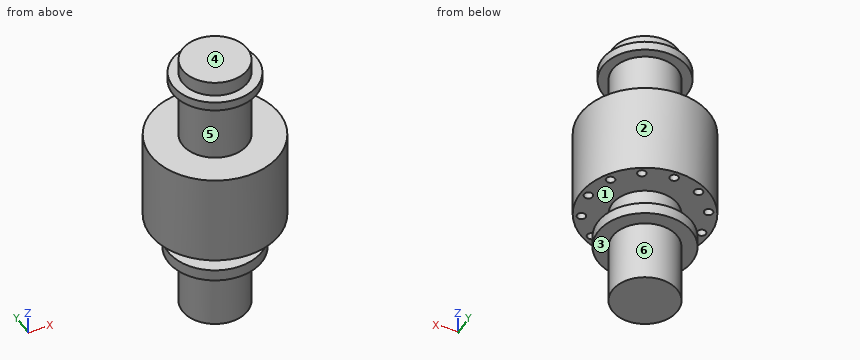
from build123d import *

# Parameters (mm, degrees)
SKETCH1_W          = 11.36904
SKETCH1_H          = 24.99995
SKETCH1_W_2        = 7.00024
SKETCH1_H_2        = 7.49935
SKETCH1_W_3        = 48.37938
SKETCH1_W_4        = 71.10476
SKETCH1_H_3        = 24.49957
SKETCH1_W_5        = 20.14982
SKETCH1_W_6        = 8.9916
SKETCH1_H_4        = 10.99947
SKETCH1_W_7        = 48.006
SKETCH2_R          = 3.3
CUT_EXTRUDE1_DEPTH = 9.525
CIRPATTERN2_COUNT  = 12


with BuildPart() as part:
    # Sketch1 → Revolve1 (revolve)
    with BuildSketch(Plane(origin=(0, 0, 0), x_dir=(0, 0, -1), z_dir=(1, 0, 0)), mode=Mode.PRIVATE) as revolve1_sk:
        with Locations((-101.8159, 12.499975)):
            Rectangle(SKETCH1_W, SKETCH1_H)
        with Locations((-92.63126, 12.499975)):
            Rectangle(SKETCH1_W_2, SKETCH1_H)
        with Locations((-92.63126, 28.749625)):
            Rectangle(SKETCH1_W_2, SKETCH1_H_2)
        with Locations((-64.94145, 12.499975)):
            Rectangle(SKETCH1_W_3, SKETCH1_H)
        with Locations((-5.19938, 12.499975)):
            Rectangle(SKETCH1_W_4, SKETCH1_H)
        with Locations((-5.19938, 37.249735)):
            Rectangle(SKETCH1_W_4, SKETCH1_H_3)
        with Locations((40.42791, 12.499975)):
            Rectangle(SKETCH1_W_5, SKETCH1_H)
        with Locations((54.99862, 12.499975)):
            Rectangle(SKETCH1_W_6, SKETCH1_H)
        with Locations((54.99862, 30.499685)):
            Rectangle(SKETCH1_W_6, SKETCH1_H_4)
        with Locations((83.49742, 12.499975)):
            Rectangle(SKETCH1_W_7, SKETCH1_H)
    revolve(revolve1_sk.sketch.rotate(Axis((0, 0, 107.50042), (0, 0, -1)), 180), axis=Axis((0, 0, 107.50042), (0, 0, -1)))

    # Sketch2 → Cut-Extrude1 (cut)
    with BuildSketch(Plane(origin=(0, 0, -30.353), x_dir=(-1, 0, 0), z_dir=(0, 0, -1))):
        with Locations(Location((0, 43.561, 0), (0, 0, 90))):
            Circle(SKETCH2_R)
    cut_extrude1 = extrude(amount=-CUT_EXTRUDE1_DEPTH, mode=Mode.SUBTRACT)

    # CirPattern2: Cut-Extrude1 ×12 about axis
    cirpattern2_axis = Axis((0, 0, 0), (0, 0, 1))
    for i in range(1, CIRPATTERN2_COUNT):
        add(cut_extrude1.rotate(cirpattern2_axis, i * 360 / CIRPATTERN2_COUNT), mode=Mode.SUBTRACT)


solid = part.part
Could you check a few things on this model? Use its own coordinates, in mm. Face numbers are marked on the shaded views. A direction names the side the tool comes from. Give positions to 0.01 mm unless a question says otherwise; leave off trailing zeros. Write each loop counter-clockwise with the first axis right and the second up, starting at its lowest first coordinate (ties: lowest second). Pieces come first, ordered by that corner, then holes. Notation, with made-up numbers: (-21, 15) -> (26, 15) arc R9 ccw to (26, 22) -> close; hole circle Ø2 at (-7.5, 84). An arc over 180 degrees is marked (long way). Answer as CSV lines item,"result". Start each with the question number.
(1) Which directions (+Z, -Z, +X, -X, +Y, -Y) give clear straight access to the entire face, cutting with the end or side of a thin tool? Please do the marked faces 4, 5 and 6.
(2) If we mould it in two halves opening along Z, with no side actions, what happens to the marked faces 1, 2 and 3? For each: +Z half, -Z half, draft (parallel to the pull), parting line (faces both ways), or undercut.
(3) Please list where these lines run through material, in increasing order: line 1 (Z direction, x = 6, y = -25.5); line 2 (X direction, y = 37, z = -28); line 3 (Z direction, x = -11, y = 40).
(4) If we section it at B-B, the plane y = 30: Write out the boundary of the cut face in (x, z).
(5) If we section it at C-C, the plane x = 7: Write out the boundary of the cut face in (y, z), and give its area (3 significant figures).
(6) I'm going to push flat-ended pins straight in: pin 1 Ø1 at (y, z) = (34.5, 23.5) entering from +X (3 decimals); pin 2 Ø3 at (y, z) = (-2.5, 21.5) entering from -X; pin 3 Ø12 at (x, z) = (-21, -32.5) entering from -Y; pin 4 Ø5 at (x, y) = (-26, 8.5) entering from +Z. Where does each tip first touch, or does it pass through?
(7) If we section it at A-A, the plane x = 29: Write out the boundary of the cut face in (y, z).
Answer list:
1,face 4,"+Z, +X, -X, +Y, -Y"
1,face 5,"none"
1,face 6,"-Z"
2,face 1,"undercut"
2,face 2,"draft"
2,face 3,"-Z half"
3,line 1,"-59.49 to -50.5, -30.35 to 40.75, 89.13 to 96.13"
3,line 2,"-32.88 to -25, -18.56 to 18.56, 25 to 32.88"
3,line 3,"-30.35 to 40.75"
4,outline,"(-39.37, -30.35) -> (39.37, -30.35) -> (39.37, 40.75) -> (-39.37, 40.75) -> close; (-19.9, -59.49) -> (19.9, -59.49) -> (19.9, -50.5) -> (-19.9, -50.5) -> close; (-12.5, 89.13) -> (12.5, 89.13) -> (12.5, 96.13) -> (-12.5, 96.13) -> close"
5,outline,"(-49, -30.35) -> (-24, -30.35) -> (-24, -50.5) -> (-35.31, -50.5) -> (-35.31, -59.49) -> (-24, -59.49) -> (-24, -107.5) -> (24, -107.5) -> (24, -59.49) -> (35.31, -59.49) -> (35.31, -50.5) -> (24, -50.5) -> (24, -30.35) -> (49, -30.35) -> (49, 40.75) -> (24, 40.75) -> (24, 89.13) -> (31.74, 89.13) -> (31.74, 96.13) -> (24, 96.13) -> (24, 107.5) -> (-24, 107.5) -> (-24, 96.13) -> (-31.74, 96.13) -> (-31.74, 89.13) -> (-24, 89.13) -> (-24, 40.75) -> (-49, 40.75) -> close"
5,area,"14,200 mm^2"
6,pin 1,"x = 35.975"
6,pin 2,"x = -49.49"
6,pin 3,"y = -47.04"
6,pin 4,"z = 107.5"
7,outline,"(-40.11, -30.35) -> (40.11, -30.35) -> (40.11, 40.75) -> (-40.11, 40.75) -> close; (-21.33, -59.49) -> (21.33, -59.49) -> (21.33, -50.5) -> (-21.33, -50.5) -> close; (-14.67, 89.13) -> (14.67, 89.13) -> (14.67, 96.13) -> (-14.67, 96.13) -> close"
